from build123d import *

# Parameters (mm, degrees)
F0_R     = 18.415
F3_DEPTH = 25.4
F1_R     = 1.4986
F4_DEPTH = 6.35
F5_DEPTH = 7.62
F7_DEPTH = 16.002


with BuildPart() as f3:
    # F0 (on Top) → F3 (new body)
    with BuildSketch(Plane.XY):
        Circle(F0_R)
    extrude(amount=F3_DEPTH)

    # F1 (on Top) → F4 (cut)
    with BuildSketch(Plane.XY):
        with Locations((-15.24, 0)):
            Circle(F1_R)
        with Locations((-7.62, -13.198227)):
            Circle(F1_R)
        with Locations((7.62, -13.198227)):
            Circle(F1_R)
        with BuildLine():
            ThreePointArc((13.7414, 0), (15.24, -1.4986), (16.7386, 0))
            ThreePointArc((16.7386, 0), (15.24, 1.4986), (13.7414, 0))
        make_face()
        with Locations((7.62, 13.198227)):
            Circle(F1_R)
        with Locations((-7.62, 13.198227)):
            Circle(F1_R)
    extrude(amount=F4_DEPTH, mode=Mode.SUBTRACT)

    # F2 (on Top) → F5 (join)
    with BuildSketch(Plane.XY):
        with BuildLine():
            ThreePointArc((0, 0.9906), (4.238681, 2.746319), (5.9944, 6.985))
            ThreePointArc((5.9944, 6.985), (-4.238681, 11.223681), (0, 0.9906))
        make_face()
    extrude(amount=-F5_DEPTH)

    # F6 (on face) → F7 (join)
    with BuildSketch(Plane(origin=(0, 0, -7.62), x_dir=(1, 0, 0), z_dir=(0, 0, -1))):
        with BuildLine():
            Line((1.840405, -4.6355), (0, -4.6355))
            Line((0, -4.6355), (-1.840405, -4.6355))
            ThreePointArc((-1.840405, -4.6355), (0, -9.9695), (1.840405, -4.6355))
        make_face()
    extrude(amount=F7_DEPTH)


solid = f3.part
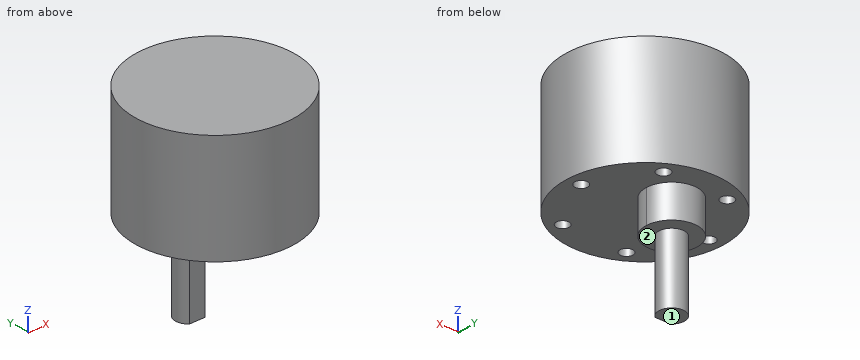
Input: part model. Units: mm. Frame: model coordinates. Face numbers are marked on the shaded views. A direction names the side the tool comes from. Coordinates: 2 decimals unless noted, no trailing zeros. Order: outer loops, then holes, each group sorted by start corner. A loop starts at its lowest first (then second) coordinate and runs counter-clockwise, first axis right, second up. Notation, with made-up numbers: M 39.5,4 L 68.5,4 A29 ccw 68.5,43 Z; hole C 79.5,-29.75 d11. An arc over 180 degrees is marked long. One line per question, with ' | ' between items.
Item 1: Section D-D (x = 15.24). Output: boundary loops of the cut face in (y, z).
Geometry results:
outline: M -10.34,0 L -1.5,0 L -1.5,6.35 L 1.5,6.35 L 1.5,0 L 10.34,0 L 10.34,25.4 L -10.34,25.4 Z
Item 2: Section B-B (x = -5). Output: boundary loops of the cut face in (y, z).
Geometry results:
outline: M -17.72,0 L 3.68,0 L 3.68,-7.62 L 10.29,-7.62 L 10.29,0 L 17.72,0 L 17.72,25.4 L -17.72,25.4 Z
Item 3: Section A-A (y = 0). Output: boundary loops of the cut face in (x, z) (3 decimals).
Geometry results:
outline: M -18.415,0 L -16.739,0 L -16.739,6.35 L -13.741,6.35 L -13.741,0 L 13.741,0 L 13.741,6.35 L 16.739,6.35 L 16.739,0 L 18.415,0 L 18.415,25.4 L -18.415,25.4 Z
Item 4: Section C-C (z = -4). Output: boundary loops of the cut face in (x, y) (3 decimals), then the cut area to 3 significant figures.
Geometry results:
outline: C 0,6.985 d11.989 | area: 113 mm^2
Item 5: Ray query, line 1 along Y through (x, z) = (7.62, 4.75); line 2 along Z through (x, y) = (8, -5); line 3 along Y through (x, z) = (0, -14.5). Return the intervals inside material, ascending.
Geometry results:
line 1: y = -16.76 to -14.7, -11.7 to 11.7, 14.7 to 16.76 | line 2: z = 0 to 25.4 | line 3: y = 4.64 to 9.97
Item 6: Reachability of the marked faces 1 and 2 from +Z, -Z, +X, -X, +Y, -Y: full face, straight path, thin tool, end or side. Return the list, or none.
Geometry results:
face 1: -Z, +X, -X, +Y, -Y | face 2: -Z
Item 7: Pin query (flat end, axial travel): pin 1 (2.5 mm diameter, centred on x = -7.62, y = -13.2, fed in from -Z); pin 2 (1 mm diameter, centred on x = 4, y = -11, fed in from -Z); pin 3 (2 mm diameter, centred on x = 9.5, z = 14.5, fed in from -Y). Return the tip coordinate at first contact, or that it passes through.
Geometry results:
pin 1: stops at z = 6.35 | pin 2: stops at z = 0 | pin 3: stops at y = -16.34
